```python
from build123d import *

# Parameters (mm, degrees)
SKETCH1_W           = 50
SKETCH1_H           = 50
BOSS_EXTRUDE1_DEPTH = 27.5
SKETCH3_R           = 22.5
BOSS_EXTRUDE2_DEPTH = 140
SKETCH4_W           = 50
SKETCH4_H           = 50
BOSS_EXTRUDE3_DEPTH = 27.5
SKETCH5_R           = 16
BOSS_EXTRUDE4_DEPTH = 15


with BuildPart() as part:
    # Sketch1 → Boss-Extrude1 (new body)
    with BuildSketch(Plane.XY):
        with Locations((25, 25)):
            Rectangle(SKETCH1_W, SKETCH1_H)
    extrude(amount=BOSS_EXTRUDE1_DEPTH)

    # Sketch3 → Boss-Extrude2 (add)
    with BuildSketch(Plane.XY.offset(27.5)):
        with Locations((25, 25)):
            Circle(SKETCH3_R)
    extrude(amount=BOSS_EXTRUDE2_DEPTH)

    # Sketch4 → Boss-Extrude3 (add)
    with BuildSketch(Plane.XY.offset(167.5)):
        with Locations((25, 25)):
            Rectangle(SKETCH4_W, SKETCH4_H)
    extrude(amount=BOSS_EXTRUDE3_DEPTH)

    # Sketch5 → Boss-Extrude4 (add)
    with BuildSketch(Plane.XY.offset(195)):
        with Locations((25, 25)):
            Circle(SKETCH5_R)
    extrude(amount=BOSS_EXTRUDE4_DEPTH)


solid = part.part
```
Work out the finished part from the listing and answer in its coordinate system (mm). A direction names the side the tool comes from. Give positions to 0.01 mm unless a question says otherwise; leave off trailing zeros. Write each loop counter-clockwise with the first axis right and the second up, starting at its lowest first coordinate (ties: lowest second). Pieces come first, ordered by that corner, then holes. Notation, with made-up numbers: (-28.75, -5.75) - (0.25, -5.75) arc R11 ccw to (0.25, 3.25) - close; hole circle Ø3 at (61, 62.25). An arc over 180 degrees is marked (long way). Use one line per item in the form item = value.
1. Determine the mould class of faces 1 (the face through (13.5, 36.5, 195)), 2 (the face through (7.145, 11.309, 96.52)), 3 (the face through (25, 0, 181)) for opening direction Y: released by +Y, released by -Y, zero draft, split by the parting line, or undercut.
Filled in:
face_1 = zero draft
face_2 = split by the parting line
face_3 = released by -Y
2. For faces 4 (the face through (25, 50, 14)), 5 (the face through (2, 25, 167.5)), 6 (the face through (21.53, 9.38, 202.4)), determine the directions among +Z, -Z, +X, -X, +Y, -Y from which every point of the face is accessible in a straight line to the end or side of a thin tool.
Filled in:
face_4 = +Z, -Z, +X, -X, +Y
face_5 = none
face_6 = +Z
3. Each of these flat-tipped pins is pushed along its axis until it touches: pin 1 Ø12 at (x, y) = (16, 28.5) entering from -Z; pin 2 Ø1.5 at (x, z) = (34, 95) entering from -Y; pin 3 Ø2 at (x, z) = (43.5, 121) entering from +Y; pin 4 Ø12 at (x, z) = (36.5, 142.5) entering from -Y. Where does it stop, or does it pass through?
Filled in:
pin_1 = 0
pin_2 = 4.07
pin_3 = 39.14
pin_4 = 3.18
4. Consider L1, parallel to Z at x = 46.5, y = 18; L2, parallel to X at y = 44.5, z = 102.5; L3, parallel to Z at x = 6, y = 30. Determine where each line is inside the solid, lowest interval first.
Filled in:
L1 = 0 to 27.5, 167.5 to 195
L2 = 13.78 to 36.22
L3 = 0 to 195
5. A cutting plane is placed at A-A (y = 25). Write down the section's boundary in (x, z).
Filled in:
outline = (0, 0) - (50, 0) - (50, 27.5) - (47.5, 27.5) - (47.5, 167.5) - (50, 167.5) - (50, 195) - (41, 195) - (41, 210) - (9, 210) - (9, 195) - (0, 195) - (0, 167.5) - (2.5, 167.5) - (2.5, 27.5) - (0, 27.5) - close
6. A cutting plane is placed at C-C (z = 46). Write down the section's boundary in (x, y), and give its area (3 significant figures).
Filled in:
outline = circle Ø45 at (25, 25)
area = 1,590 mm^2
